Design review of the part shown in the three views and the two pictorial views. Dimensions are in mm from the part's minimum x, y and z. A direction names the side the tool comes from. Coordinates: 2 decimals unless noted, no trailing zeros. Order: outer loops, then holes, each group sorted by start corner. A loop starts at its lowest first (then second) coordinate and runs counter-clockwise, first axis right, second up. Notation, with made-up numbers: (76.25, 87.25) - (127.25, 87.25) arc R17 cw to (127.25, 108.25) - close; hole circle Ø8 at (26.25, 3). An arc over 180 degrees is marked (long way). One line per item, written item: value. Start each with the question number.
(1) Consider section A-A on z = 9.75. Count the separate pieces of the cut face and the enclosed holes in it, then the cut area to 3 significant figures.
(2) Consider section B-B on x = 9. Write out the cut boundary in (y, z) (1 decimal).
(3) Clearance check with flat-ended pins moving along their axes: pin 1 (5 mm diameter, centred on y = 62, z = 9.5, fed in from -X) (1 decimal); pin 2 (5.5 mm diameter, centred on x = 87.5, z = 10, fed in from -Y); pin 3 (8 mm diameter, centred on x = 7, z = 10, fed in from +Y); pin 4 (6 mm diameter, centred on x = 87.31, z = 7.94, fed in from +Y). State where each tip first meets the part, or that it passes through.
(4) Mouldability with a two-part tool opening along X and no side actions: class the marked faces 6, 7 and 8 as released by +X, released by -X, zero draft, split by the parting line, or undercut.
(5) To check wall thickness, follow line 1 along X through (y, z) = (16.5, 10); line 2 along X through (y, z) = (54, 3) (1 decimal); line 3 along Y through (x, z) = (87, 3.25) (1 decimal). State the ranges of each line that lie inside material, in increasing order.
(6) For the marked faces 1, 2, 3, 4 and 5, list the 3-axis set-ups (+Z, -Z, +X, -X, +Y, -Y) from which the entire face can be reached by the end or side of a thin tool; tool diameter is ignored.
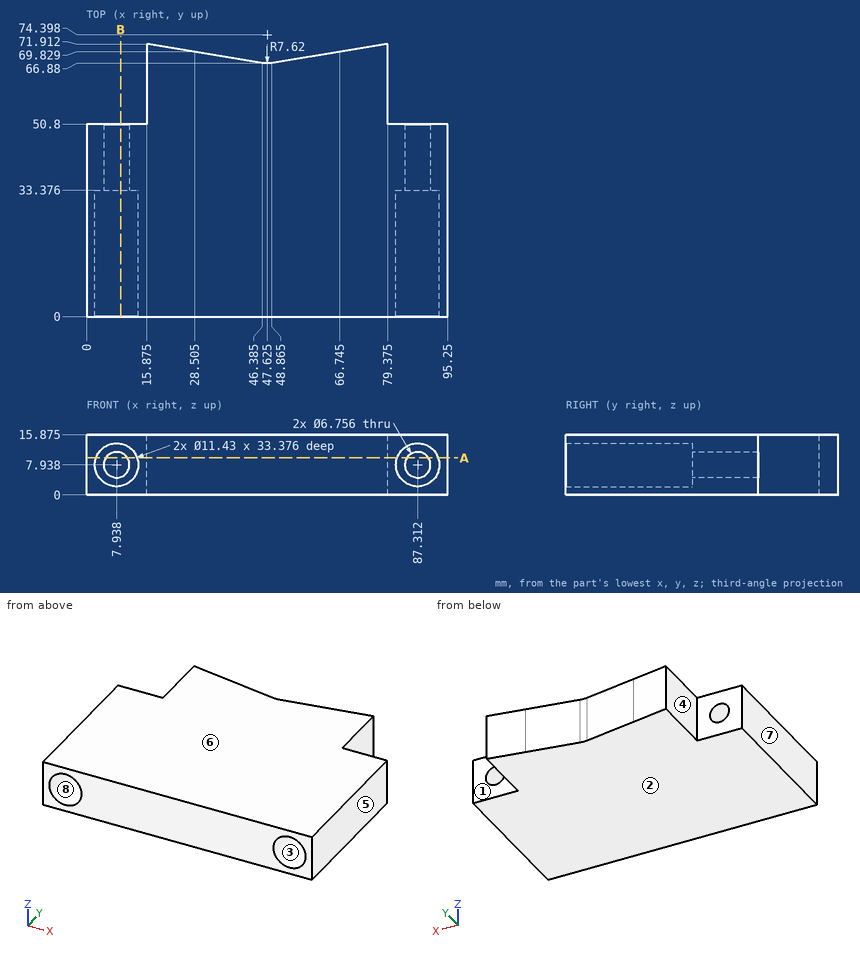
Geometry check:
1. separate pieces: 3
1. enclosed holes: 0
1. area: 5,090 mm^2
2. outline: (0, 0) - (50.8, 0) - (50.8, 4.7) - (33.4, 4.7) - (33.4, 2.3) - (0, 2.3) - close; (0, 13.6) - (33.4, 13.6) - (33.4, 11.1) - (50.8, 11.1) - (50.8, 15.9) - (0, 15.9) - close
3. pin 1: stops at x = 15.9
3. pin 2: stops at y = 33.38
3. pin 3: stops at y = 50.8
3. pin 4: passes through
4. face 6: zero draft
4. face 7: released by -X
4. face 8: undercut
5. line 1: x = 0 to 2.61, 13.27 to 81.98, 92.64 to 95.25
5. line 2: x = 15.9 to 79.4
5. line 3: y = 33.4 to 50.8
6. face 1: +Z, -Z, +X, +Y
6. face 2: -Z, +X, -X, +Y, -Y
6. face 3: -Y
6. face 4: +Z, -Z, -X, +Y
6. face 5: +Z, -Z, +X, +Y, -Y
